Geometry: final body of the model. Coordinates: model frame, mm. Give positions to 0.01 mm unless a question says otherwise; leave off trailing zeros. Write each loop counter-clockwise with the first axis right and the second up, starting at its lowest first coordinate (ties: lowest second). Pieces come first, ordered by that corner, then holes.
Q1. Section C-C (z = 2.85). Return the cut outline in (x, y).
Q2. Section B-B (y = 59.5). Return the cut outline in (x, z).
Q3. Section D-D (y = 34.5). Return the cut outline in (x, z).
Q4. Pin query (flat end, axial travel): pin 1 Ø0.8 at (x, z) = (31, 1.5) entering from +Y; pin 2 Ø1.1 at (x, y) = (-42, 72) entering from -Z; pin 3 Ø6 at (x, y) = (-35.5, 50) entering from +Z; pin 4 Ø0.5 at (x, z) = (-44, 1.5) entering from -Y. Return the tip coordinate at first contact, or that it passes through.
Q5. Line query: line 1 (Z direction, x = -20.5, y = 72); line 2 (Y direction, x = 2, z = 5.1); line 3 (Y direction, x = 13, z = 3.35). Output: solid intervals per line, ascending.
Q6. Section A-A (x = -15). Return the cut outline in (y, z), plus the area to 3 significant figures.
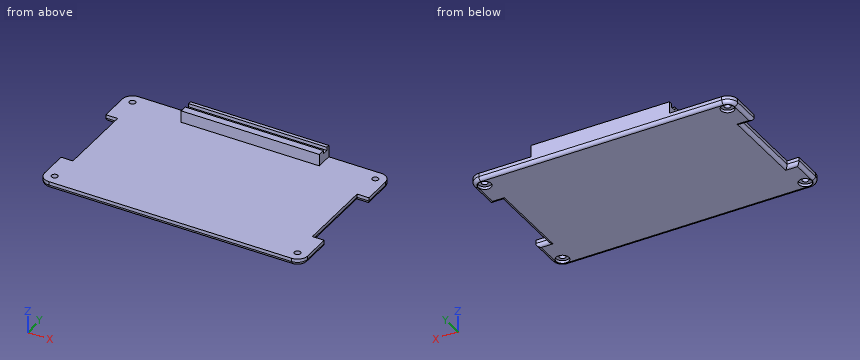
from build123d import *

# Parameters (mm, degrees)
F1_DEPTH  = 2
F2_R      = 3
F3_R      = 0.9
F4_DEPTH  = 2.5
F5_R      = 1
F6_W      = 40.96
F6_H      = 4.9
F7_DEPTH  = 3.5
F8_W      = 40.96
F8_H      = 1.8
F9_DEPTH  = 1
F10_ANGLE = 180
F12_R     = 1.9
F13_DEPTH = 0.8


with BuildPart() as f1:
    # F0 (on Top) → F1 (new body)
    with BuildSketch(Plane.XY):
        Polygon((33.1217415035, 28.7645919905), (-44.8782584965, 28.7645919905), (-44.8782584965, 17.2645919905), (-41.3782584965, 17.2645919905), (-41.3782584965, -5.7354080095), (-44.8782584965, -5.7354080095), (-44.8782584965, -17.2354080095), (33.1217415035, -17.2354080095), (33.1217415035, -5.7354080095), (29.6217415035, -5.7354080095), (29.6217415035, 17.2645919905), (33.1217415035, 17.2645919905), align=None)
    extrude(amount=F1_DEPTH)

    # F2
    f2_edges = [f1.edges().sort_by_distance(p)[0] for p in [
        (-44.878258, 28.764592, 1),
        (33.121742, 28.764592, 1),
        (33.121742, -17.235408, 1),
        (-44.878258, -17.235408, 1),
    ]]
    fillet(f2_edges, radius=F2_R)

    # F3 (on face) → F4 (cut)
    with BuildSketch(Plane.XY.offset(2)):
        with Locations((-41.8782584965, -14.2354080095)):
            Circle(F3_R)
        with Locations((30.1217415035, -14.2354080095)):
            Circle(F3_R)
        with Locations((30.1217415035, 25.7645919905)):
            Circle(F3_R)
        with Locations((-41.8782584965, 25.7645919905)):
            Circle(F3_R)
    extrude(amount=-F4_DEPTH, mode=Mode.SUBTRACT)

    # F5
    f5_edges = [f1.edges().sort_by_distance(p)[0] for p in [
        (33.121742, -9.985408, 2),
        (32.243062, -16.356728, 2),
        (31.371742, -5.735408, 2),
        (29.621742, 5.764592, 2),
        (31.371742, 17.264592, 2),
        (33.121742, 21.514592, 2),
        (-43.128258, 17.264592, 2),
        (-41.378258, 5.764592, 2),
        (-43.128258, -5.735408, 2),
    ]]
    fillet(f5_edges, radius=F5_R)

    # F6 (on face) → F7 (join)
    with BuildSketch(Plane(origin=(0, 0, 0), x_dir=(1, 0, 0), z_dir=(0, 0, -1))):
        with Locations((-5.8782584965, 14.7854080095)):
            Rectangle(F6_W, F6_H)
    extrude(amount=F7_DEPTH)

    # F8 (on face) → F9 (cut)
    with BuildSketch(Plane(origin=(0, 0, -3.5), x_dir=(1, 0, 0), z_dir=(0, 0, -1))):
        with Locations((-5.8782584965, 15.3354080095)):
            Rectangle(F8_W, F8_H)
    extrude(amount=-F9_DEPTH, mode=Mode.SUBTRACT)


with BuildPart() as f1_1:
    # F10: moved
    add(f1.part.rotate(Axis((-5.8782584965, 28.7645919905, 0), (1, 0, 0)), F10_ANGLE))


with BuildPart() as f1_2:
    # F11: moved
    add(f1_1.part.moved(Location((0, 0, 2))))

    # F12 (on face) → F13 (cut)
    with BuildSketch(Plane(origin=(0, 0, 0), x_dir=(1, 0, 0), z_dir=(0, 0, -1))):
        with Locations((-41.8782584965, -31.7645919905)):
            Circle(F12_R)
        with Locations((-41.8782584965, -71.7645919905)):
            Circle(F12_R)
        with Locations((30.1217415035, -71.7645919905)):
            Circle(F12_R)
        with Locations((30.1217415035, -31.7645919905)):
            Circle(F12_R)
    extrude(amount=-F13_DEPTH, mode=Mode.SUBTRACT)


solid = f1_2.part
Computed:
1. outline: (-26.36, 69.86) - (14.6, 69.86) - (14.6, 74.76) - (-26.36, 74.76) - close
2. outline: (-41.38, 1) arc R1 ccw to (-40.38, 0) - (28.62, 0) arc R1 ccw to (29.62, 1) - (29.62, 2) - (-41.38, 2) - close
3. outline: (-44.88, 1) arc R1 ccw to (-43.88, 0) - (32.12, 0) arc R1 ccw to (33.12, 1) - (33.12, 2) - (-44.88, 2) - close
4. pin 1: stops at y = 74.73
4. pin 2: passes through
4. pin 3: stops at z = 2
4. pin 4: stops at y = 29.42
5. line 1: z = 0 to 4.5
5. line 2: y = 69.86 to 71.96, 73.76 to 74.76
5. line 3: y = 69.86 to 74.76
6. outline: (28.76, 1) arc R1 ccw to (29.76, 0) - (73.76, 0) arc R1 ccw to (74.76, 1) - (74.76, 5.5) - (73.76, 5.5) - (73.76, 4.5) - (71.96, 4.5) - (71.96, 5.5) - (69.86, 5.5) - (69.86, 2) - (28.76, 2) - close
6. area: 107 mm2
